```python
from build123d import *

# Parameters (mm, degrees)
BOSS_EXTRUDE1_DEPTH = 3.81
SKETCH2_R           = 3.175
CUT_EXTRUDE1_DEPTH  = 434.546807932


with BuildPart() as part:
    # Sketch1 → Boss-Extrude1 (new body)
    with BuildSketch(Plane.XY):
        with BuildLine():
            Line((70.358, 337.34375), (70.358, 388.14375))
            ThreePointArc((70.358, 388.14375), (71.586192113, 399.190379334), (75.210780547, 409.697464286))
            ThreePointArc((75.210780547, 409.697464286), (74.514154695, 421.194879412), (64.424703202, 426.75175))
            Line((64.424703202, 426.75175), (-64.424703202, 426.75175))
            ThreePointArc((-64.424703202, 426.75175), (-74.514154695, 421.194879412), (-75.210780547, 409.697464286))
            ThreePointArc((-75.210780547, 409.697464286), (-71.586192113, 399.190379334), (-70.358, 388.14375))
            Line((-70.358, 388.14375), (-70.358, 337.34375))
            ThreePointArc((-70.358, 337.34375), (-70.425674666, 334.735607232), (-70.628516531, 332.134483679))
            ThreePointArc((-70.628516531, 332.134483679), (-66.887034969, 322.158291888), (-56.667646584, 319.143795582))
            ThreePointArc((-56.667646584, 319.143795582), (0, 324.13575), (56.667646584, 319.143795582))
            ThreePointArc((56.667646584, 319.143795582), (66.887034969, 322.158291888), (70.628516531, 332.134483679))
            ThreePointArc((70.628516531, 332.134483679), (70.425674666, 334.735607232), (70.358, 337.34375))
        make_face()
    extrude(amount=BOSS_EXTRUDE1_DEPTH)

    # Sketch2 → Cut-Extrude1 (cut, through all)
    with BuildSketch(Plane.XY.offset(3.81)):
        with Locations((-19.05, 332.89875)):
            Circle(SKETCH2_R)
        with Locations((0, 332.89875)):
            Circle(SKETCH2_R)
        with Locations((19.05, 332.89875)):
            Circle(SKETCH2_R)
        with BuildLine():
            Line((-52.705, 420.40175), (52.705, 420.40175))
            ThreePointArc((52.705, 420.40175), (53.603025612, 420.029775612), (53.975, 419.13175))
            Line((53.975, 419.13175), (53.975, 343.69375))
            ThreePointArc((53.975, 343.69375), (53.603025612, 342.795724388), (52.705, 342.42375))
            Line((52.705, 342.42375), (-52.705, 342.42375))
            ThreePointArc((-52.705, 342.42375), (-53.603025612, 342.795724388), (-53.975, 343.69375))
            Line((-53.975, 343.69375), (-53.975, 419.13175))
            ThreePointArc((-53.975, 419.13175), (-53.603025612, 420.029775612), (-52.705, 420.40175))
        make_face()
    extrude(amount=-CUT_EXTRUDE1_DEPTH, mode=Mode.SUBTRACT)


solid = part.part
```
Geometry: final body of the model. Coordinates: model frame, mm. A direction names the side the tool comes from. Round coordinates to 2 decimals unless told otherwise and drop trailing zeros. Loops run counter-clockwise (first coordinate to the right, second up) from the corner with the lowest first, then second, coordinate; pieces in that order, holes last. Notation, with made-up numbers: (65, -30.75) -> (92, -30.75) arc R11 ccw to (92, -21.75) -> close; hole circle Ø6 at (18.5, 84). An arc over 180 degrees is marked (long way). Write each question's results on one line, items separated by ' | '.
Item 1: Pull-direction query (X, two-part tool) for faces 1 (the face through (1, 426.752, 2)), 2 (the face through (-71.62, 399.34, 1.88)), 3 (the face through (53.975, 382, 2)), 4 (the face through (-53.975, 381, 2)); classes: pulls with the +X half, pulls with the -X half, needs draft (parallel to the pull), parting line crosses it, or undercut.
Answers below:
face 1: needs draft | face 2: pulls with the -X half | face 3: undercut | face 4: undercut
Item 2: Cut plane C-C on z = 1.6. State how many separate pieces and enclosed holes the cut face has, and give its area (3 significant figures).
Answers below:
separate pieces: 1 | enclosed holes: 4 | area: 6,410 mm²
Item 3: Cut plane D-D on y = 395. Return the cut outline in (x, z) (3 decimals), and give its area (3 significant figures).
Answers below:
outline: (-70.828, 0) -> (-53.975, 0) -> (-53.975, 3.81) -> (-70.828, 3.81) -> close; (53.975, 0) -> (70.828, 0) -> (70.828, 3.81) -> (53.975, 3.81) -> close | area: 128 mm²
Item 4: Set-up query: faces 5 (the face through (-1, 420.402, 2)), 6 (the face through (-0.797, 324.135, 1.878)), 7 (the face through (70.428, 334.699, 1.878)), 8 (the face through (-1, 338, 0)), 9 (the face through (-70.358, 363, 2)). Return all of +Z, -Z, +X, -X, +Y, -Y with unobstructed straight access to the full face (end or side cutting, diameter ignored); none if empty.
Answers below:
face 5: +Z, -Z | face 6: +Z, -Z, -Y | face 7: +Z, -Z, +X | face 8: -Z, +X, -X, +Y, -Y | face 9: +Z, -Z, -X
Item 5: Cut plane A-A on x = 0. Return the cut outline in (y, z).
Answers below:
outline: (324.14, 0) -> (329.72, 0) -> (329.72, 3.81) -> (324.14, 3.81) -> close; (336.07, 0) -> (342.42, 0) -> (342.42, 3.81) -> (336.07, 3.81) -> close; (420.4, 0) -> (426.75, 0) -> (426.75, 3.81) -> (420.4, 3.81) -> close
Item 6: Cut plane B-B on y = 361.5. Return the cut outline in (x, z) (3 decimals).
Answers below:
outline: (-70.358, 0) -> (-53.975, 0) -> (-53.975, 3.81) -> (-70.358, 3.81) -> close; (53.975, 0) -> (70.358, 0) -> (70.358, 3.81) -> (53.975, 3.81) -> close
Item 7: Pin query (flat end, axial travel): pin 1 Ø1.9 at (y, z) = (364.5, 2.5) entering from -X; pin 2 Ø1.1 at (y, z) = (354.5, 2.5) entering from +X; pin 3 Ø2 at (y, z) = (410, 1.5) entering from +X. Return the tip coordinate at first contact, or that it passes through.
Answers below:
pin 1: stops at x = -70.36 | pin 2: stops at x = 70.36 | pin 3: stops at x = 75.74
Item 8: Line query: probe 1 along X at (y, z) = (393, 2.85) (3 decimals); probe 2 along X at (y, z) = (414, 1.15) (3 decimals); probe 3 along Y at (x, z) = (19.05, 1.7). Output: solid intervals per line, ascending. Write a range as [from, to].
Answers below:
probe 1: x = [-70.593, -53.975], [53.975, 70.593] | probe 2: x = [-76.335, -53.975], [53.975, 76.335] | probe 3: y = [323.58, 329.72], [336.07, 342.42], [420.4, 426.75]
